Can you work these out from the model? Positions are in its coordinate system, mm. Face numbers are marked on the shaded views. Round coordinates to 2 decimals unless told otherwise and drop trailing zeros. Write each loop counter-clockwise with the first axis right and the second up, starting at its lowest first coordinate (ties: lowest second). Pieces come first, ordered by that corner, then holes. Notation, with made-up numbers: (-3, -4) - (19, -4) arc R27 ccw to (19, 31) - close; hole circle Ø3 at (57.5, 69.5). An arc over 180 degrees is marked (long way). One line per item, written item: value. Start each with the question number.
(1) Thinking about a two-plate mould opening in Y: for the marked faces 1, 2 and 3, which applies, +Y half, -Y half, draft (parallel to the pull), parting line (faces both ways), or undercut?
(2) If I drill on L1, parallel to Y at x = 5.5, z = -0.25; L2, parallel to Y at x = -3.5, z = 0.5; L3, parallel to X at y = 83, z = -4, over which ranges is the centre line in solid material (lowest first)? Write a range as from..to.
(3) I want a section at A-A on y = 15.5. List the corners of the cut face in (x, z) for me, plus the area to 3 significant figures.
(4) I'm going to push flat-ended pins straight in: pin 1 Ø2 at (y, z) = (76, -0.5) entering from +X; pin 2 Ø8 at (x, y) = (-4, 80.5) entering from -Z; pin 3 Ø1.5 at (y, z) = (137.5, 3.5) entering from +X. Where does each tip first touch, or does it pass through?
Autodesk Inventor part; units mm, degrees
ref_plane "Work Plane1" through (-5, 0, 0) normal (1, 0, 0) x (0, 1, 0)
ref_plane "Work Plane4" through (0, 33, 0) normal (0, -1, 0) x (1, 0, 0)
ref_plane "Work Plane5" through (0, 165, 0) normal (0, 1, 0) x (1, 0, 0)
sketch "Sketch1" plane through (0, 0, 0) normal (0, 1, 0) x (-1, 0, 0)
  circle A0 centre (0, 0) radius 5
  point P0 (0, 5)
  dimension "d0" = 10
extrude "Extrusion1" add sketch "Sketch1" along normal blind 180
ref_plane "Work Plane1" through (-5, 0, 0) normal (1, 0, 0) x (0, 1, 0)
ref_plane "Work Plane4" through (0, 33, 0) normal (0, -1, 0) x (1, 0, 0)
sketch "Sketch7" plane through (0, 33, 0) normal (0, -1, 0) x (1, 0, 0)
  circle A0 centre (0, 0) radius 7
  dimension "d29" = 14
extrude "Extrusion7" add sketch "Sketch7" along normal blind 4
ref_plane "Work Plane5" through (0, 165, 0) normal (0, 1, 0) x (1, 0, 0)
sketch "Sketch8" plane through (0, 165, 0) normal (0, 1, 0) x (1, 0, 0)
  circle A0 centre (0, 0) radius 7
  dimension "d33" = 14
extrude "Extrusion8" add sketch "Sketch8" along normal blind 4
sketch "Sketch2" plane through (-5, 0, 0) normal (1, 0, 0) x (0, 1, 0)
  line L0 (150, -1) -> (130, -1)
  line L1 (130, -1) -> (130, 1)
  line L2 (130, 1) -> (150, 1)
  line L3 (150, 1) -> (150, -1)
  line L4 (150, 0) -> (130, 0) construction
  line L5 (180, -5) -> (180, 5) construction
  line L6 (180, 0) -> (0, 0) construction
  line L7 (0, 5) -> (0, -5) construction
  line L8 (70, -1) -> (50, -1)
  line L9 (50, -1) -> (50, 1)
  line L10 (50, 1) -> (70, 1)
  line L11 (70, 1) -> (70, -1)
  line L12 (70, 0) -> (50, 0) construction
  line L13 (165, 7) -> (165, -7)
  line L14 (33, -7) -> (33, 7)
  line L15 (169, -7) -> (169, 7)
  dimension "d3" = 20
  dimension "d4" = 2
  dimension "d6" = 20
  dimension "d7" = 2
  dimension "d36" = 15
  dimension "d37" = 17
  dimension "d38" = 60
  dimension "d40" = 15
  dimension "d41" = 33
extrude "Extrusion2" cut sketch "Sketch2" along normal blind 2
pattern_circular "Circular Pattern1" count 4 over 360 about axis through (0, -10, 0) along (0, 1, 0) of "Extrusion2"
sketch "Sketch9" plane through (0, 180, 0) normal (0, 1, 0) x (1, 0, 0)
  circle A0 centre (0, 0) radius 5
  dimension "d42" = 10
extrude "Extrusion9" cut sketch "Sketch9" against normal blind 9
properties part number "middleRod" material "Aluminum 6061"
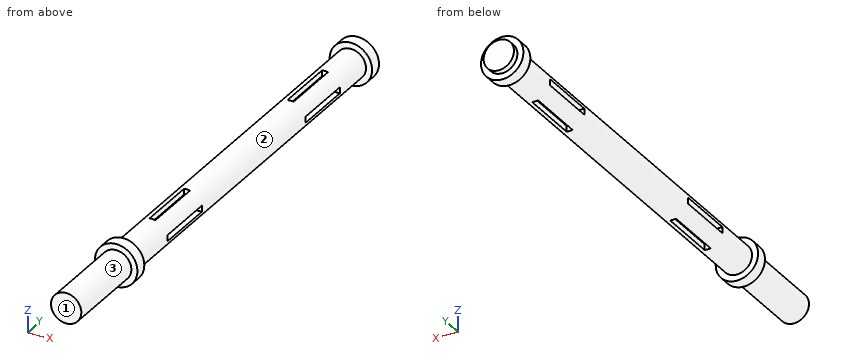
Established:
1. face 1: -Y half
1. face 2: undercut
1. face 3: draft
2. L1: 29..33, 165..169
2. L2: 0..50, 70..130, 150..171
2. L3: -3..3
3. outline: circle Ø10 at (0, 0)
3. area: 78.5 mm2
4. pin 1: x = 5
4. pin 2: z = -5
4. pin 3: x = 4.18
